The model under review builds one solid part; all positions refer to its coordinate system, in mm. Round coordinates to 2 decimals unless told otherwise and drop trailing zeros. Write each loop counter-clockwise with the first axis right and the second up, starting at its lowest first coordinate (ties: lowest second). Pieces come first, ordered by that corner, then holes. Notation, with made-up numbers: (67.25, -27) -> (104.25, -27) arc R13 cw to (104.25, -5) -> close; hole circle Ø8 at (0, -31). An arc over 180 degrees is marked (long way). Return JSON: item names as keys, results as strings. Group by question number.
1. Mouldability with a two-part tool opening along X and no side actions: class faces 1 (the flat face through (8.5, -153, 6)), 2 (the flat face through (0, -153, 10)), 3 (the flat face through (10, -153, -7)) as pulls with the +X half, pulls with the -X half, needs draft (parallel to the pull), parting line crosses it, or undercut.
2. Take a section at A-A, the plane x = -3. Write out the cut boundary in (y, z).
3. Take a section at B-B, the plane y = -22.5. Write out the cut boundary in (x, z), then the cut area to 3 significant figures.
4. For line 1 along Z through (x, y) = (-0.25, -251.5); line 2 along X through (y, z) = (-303.5, 6), list the stretches that pass through material, from the lowest coordinate up. Write a range as from..to.
5. Clearance check with flat-ended pins moving along their axes: P1, Ø8, axis at y = -51, z = -5, coming from the +X side; P2, Ø1, axis at x = 3.5, z = -7.5, coming from the +Y side. State where each tip first meets the part, or that it passes through.
from build123d import *

# Parameters (mm, degrees)
BOSS_EXTRUDE1_START           = 11.873397
SKETCH2_W                     = 20
SKETCH2_H                     = 20
SKETCH2_W_2                   = 17
SKETCH2_H_2                   = 17
BOSS_EXTRUDE1_DEPTH           = 335.093577
M4_CLEARANCE_HOLE1_AT_2_COUNT = 2
M4_CLEARANCE_HOLE1_AT_2_PITCH = 12
M4_CLEARANCE_HOLE2_AT_2_COUNT = 2
M4_CLEARANCE_HOLE2_AT_2_PITCH = 12
M4_CLEARANCE_HOLE3_AT_2_COUNT = 2
M4_CLEARANCE_HOLE3_AT_2_PITCH = 14.999999999
M4_CLEARANCE_HOLE4_AT_2_COUNT = 2
M4_CLEARANCE_HOLE4_AT_2_PITCH = 14.999999999
CUT_EXTRUDE1_DEPTH            = 324.529418692
CUT_EXTRUDE1_DEPTH_BACK       = 324.529418692


with BuildPart() as part:
    # Sketch2 → Boss-Extrude1 (new body)
    with BuildSketch(Plane(origin=(0, 0, 0), x_dir=(1, 0, 0), z_dir=(0, 1, 0)).offset(BOSS_EXTRUDE1_START)):
        Rectangle(SKETCH2_W, SKETCH2_H)
        Rectangle(SKETCH2_W_2, SKETCH2_H_2, mode=Mode.SUBTRACT)
    extrude(amount=-BOSS_EXTRUDE1_DEPTH)

    # Sketch5 → M4 Clearance Hole1 (revolve, cut)
    with BuildSketch(Plane(origin=(-10, 4.873397172, 3.5), x_dir=(0, 0, 1), z_dir=(0, 1, 0))):
        Polygon((0, 0), (0, 1.5), (2.15, 1.5), (2.15, 0.025), (2.175, 0), align=None)
    m4_clearance_hole1 = revolve(axis=Axis((-16.35, 4.873397172, 3.5), (1, 0, 0)), mode=Mode.SUBTRACT)

    # M4 Clearance Hole1 at 2: M4 Clearance Hole1 ×2
    with Locations(*[Vector(0, -0.8122328620674136, -0.5833333333333335) * (i * M4_CLEARANCE_HOLE1_AT_2_PITCH) for i in range(1, M4_CLEARANCE_HOLE1_AT_2_COUNT)]):
        add(m4_clearance_hole1, mode=Mode.SUBTRACT)

    # Sketch8 → M4 Clearance Hole2 (revolve, cut)
    with BuildSketch(Plane(origin=(10, 4.873397172, -3.5), x_dir=(0, 0, -1), z_dir=(0, 1, 0))):
        Polygon((0, 0), (0, 1.5), (2.15, 1.5), (2.15, 0.025), (2.175, 0), align=None)
    m4_clearance_hole2 = revolve(axis=Axis((16.35, 4.873397172, -3.5), (-1, 0, 0)), mode=Mode.SUBTRACT)

    # M4 Clearance Hole2 at 2: M4 Clearance Hole2 ×2
    with Locations(*[Vector(0, -0.8122328620674134, 0.5833333333333337) * (i * M4_CLEARANCE_HOLE2_AT_2_PITCH) for i in range(1, M4_CLEARANCE_HOLE2_AT_2_COUNT)]):
        add(m4_clearance_hole2, mode=Mode.SUBTRACT)

    # Sketch10 → M4 Clearance Hole3 (revolve, cut)
    with BuildSketch(Plane(origin=(-10, -304.720180379, -4.5), x_dir=(0, 0, 1), z_dir=(0, 1, 0))):
        Polygon((0, 0), (0, 1.5), (2.15, 1.5), (2.15, 0.025), (2.175, 0), align=None)
    m4_clearance_hole3 = revolve(axis=Axis((-16.35, -304.720180379, -4.5), (1, 0, 0)), mode=Mode.SUBTRACT)

    # M4 Clearance Hole3 at 2: M4 Clearance Hole3 ×2
    with Locations(*[Vector(0, -0.7999999999715266, 0.6000000000379647) * (i * M4_CLEARANCE_HOLE3_AT_2_PITCH) for i in range(1, M4_CLEARANCE_HOLE3_AT_2_COUNT)]):
        add(m4_clearance_hole3, mode=Mode.SUBTRACT)

    # Sketch12 → M4 Clearance Hole4 (revolve, cut)
    with BuildSketch(Plane(origin=(10, -304.720180379, 4.5), x_dir=(0, 0, -1), z_dir=(0, 1, 0))):
        Polygon((0, 0), (0, 1.5), (2.15, 1.5), (2.15, 0.025), (2.175, 0), align=None)
    m4_clearance_hole4 = revolve(axis=Axis((16.35, -304.720180379, 4.5), (-1, 0, 0)), mode=Mode.SUBTRACT)

    # M4 Clearance Hole4 at 2: M4 Clearance Hole4 ×2
    with Locations(*[Vector(0, -0.7999999999715265, -0.6000000000379647) * (i * M4_CLEARANCE_HOLE4_AT_2_PITCH) for i in range(1, M4_CLEARANCE_HOLE4_AT_2_COUNT)]):
        add(m4_clearance_hole4, mode=Mode.SUBTRACT)

    # Sketch13 → Cut-Extrude1 (cut, two sides: drawn at the far end of the back side and taken through both)
    with BuildSketch(Plane(origin=(0, 0, 0), x_dir=(0, 0, -1), z_dir=(1, 0, 0)).offset(-CUT_EXTRUDE1_DEPTH_BACK)):
        Polygon((6.5, -279.677709563), (-4.611616577, -295.220180379), (6.5, -295.220180379), align=None)
        Polygon((-6.5, -255.898810962), (6.04145572, -273.441281778), (-6.5, -290.983752595), align=None)
        Polygon((6.5, -232.119912362), (-6.04145572, -249.662383178), (6.5, -267.204853994), align=None)
        Polygon((-6.5, -208.341013761), (6.04145572, -225.883484577), (-6.5, -243.425955393), align=None)
        Polygon((6.5, -184.56211516), (-6.04145572, -202.104585977), (6.5, -219.647056793), align=None)
        Polygon((-6.5, -160.78321656), (6.04145572, -178.325687376), (-6.5, -195.868158192), align=None)
        Polygon((6.5, -137.004317959), (-6.04145572, -154.546788776), (6.5, -172.089259592), align=None)
        Polygon((-6.5, -113.225419359), (6.04145572, -130.767890175), (-6.5, -148.310360991), align=None)
        Polygon((6.5, -89.446520758), (-6.04145572, -106.988991575), (6.5, -124.531462391), align=None)
        Polygon((-6.5, -65.667622158), (6.04145572, -83.210092974), (-6.5, -100.75256379), align=None)
        Polygon((-6.04145572, -59.431194373), (6.5, -76.97366519), (6.5, -41.888723557), align=None)
        Polygon((-6.5, -18.109824957), (6.04145572, -35.652295773), (-6.5, -53.194766589), align=None)
        Polygon((6.5, -13.873397172), (6.5, -29.415867989), (-4.611616577, -13.873397172), align=None)
    extrude(amount=CUT_EXTRUDE1_DEPTH + CUT_EXTRUDE1_DEPTH_BACK, mode=Mode.SUBTRACT)


solid = part.part
Output:
{
 "1": {"face 1": "undercut", "face 2": "needs draft", "face 3": "pulls with the +X half"},
 "2": {"outline": "(-323.22, -10) -> (11.87, -10) -> (11.87, -8.5) -> (-323.22, -8.5) -> close; (-323.22, 8.5) -> (11.87, 8.5) -> (11.87, 10) -> (-323.22, 10) -> close"},
 "3": {"outline": "(-10, -10) -> (10, -10) -> (10, -6.5) -> (8.5, -6.5) -> (8.5, -8.5) -> (-8.5, -8.5) -> (-8.5, -6.5) -> (-10, -6.5) -> close; (-10, -1.56) -> (-8.5, -1.56) -> (-8.5, 3.36) -> (-10, 3.36) -> close; (-10, 6.5) -> (-8.5, 6.5) -> (-8.5, 8.5) -> (8.5, 8.5) -> (8.5, 6.5) -> (10, 6.5) -> (10, 10) -> (-10, 10) -> close; (8.5, -1.56) -> (10, -1.56) -> (10, 3.36) -> (8.5, 3.36) -> close", "area": "86.8 mm^2"},
 "4": {"line 1": "z = -10..-8.5, 8.5..10", "line 2": "x = -10..-8.5"},
 "5": {"P1": "stops at x = 10", "P2": "passes through"}
}
